Could you check a few things on this drawing? It's one solid part, dimensions in mm from its lowest x, y, z. A direction names the side the tool comes from. Coordinates: 2 decimals unless noted, no trailing zeros. Write each loop counter-clockwise with the first axis right and the second up, starting at its lowest first coordinate (ties: lowest second). Pieces come first, ordered by that corner, then holes. Notation, with made-up numbers: M -25,61 L 7,61 A15 ccw 7,85 Z; hole C -13.75,-22 d11. An arc over 180 degrees is marked long. Use a Markdown table: item, result.
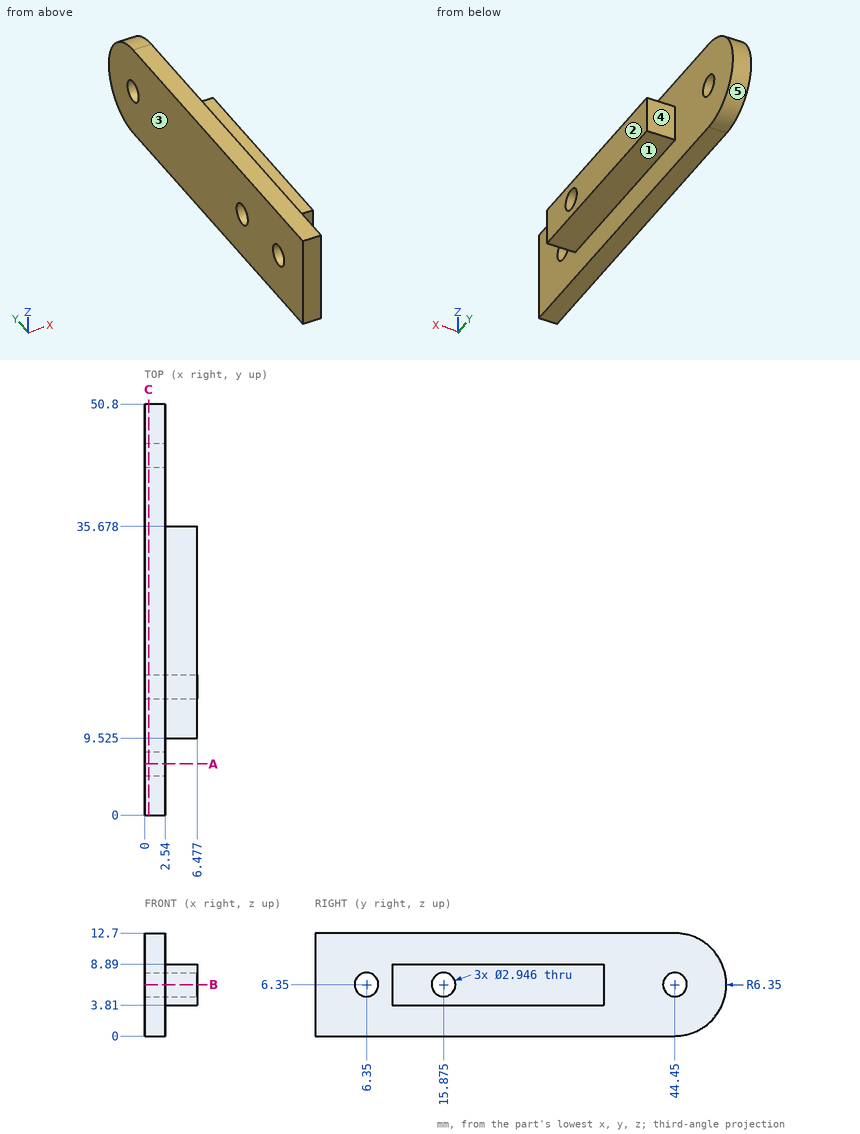
1. Which directions (+Z, -Z, +X, -X, +Y, -Y) give clear straight access to the entire face, cutting with the end or side of a thin tool? Please do the marked faces 4 and 5.
Answers follow:
| item | result |
|---|---|
| face 4 | +Z, -Z, +X, +Y |
| face 5 | +X, -X, +Y |
2. Will these pins go through, and if not, where does the flat tip stop? pin 1 Ø3 at (y, z) = (37.5, 9) entering from +X; pin 2 Ø2.5 at (y, z) = (15.875, 6.35) entering from +X; pin 3 Ø3 at (x, y) = (5, 22) entering from +Z; pin 4 Ø1.5 at (x, z) = (1, 5) entering from -Y.
Answers follow:
| item | result |
|---|---|
| pin 1 | stops at x = 2.54 |
| pin 2 | passes through |
| pin 3 | stops at z = 8.89 |
| pin 4 | stops at y = 0 |
3. I need wall thicknesses on probe 1 along Y at (x, z) = (0.8, 6.35); probe 2 along Y at (x, z) = (4.75, 6.35) (1 decimal); probe 3 along Z at (x, y) = (5, 18). Which ranges of each line are inside material? Lowest first, please.
Answers follow:
| item | result |
|---|---|
| probe 1 | y = 0 to 4.88, 7.82 to 14.4, 17.35 to 42.98, 45.92 to 50.8 |
| probe 2 | y = 9.5 to 14.4, 17.3 to 35.7 |
| probe 3 | z = 3.81 to 8.89 |
4. We'd pull the mould along X, two halves only. Please class the marked faces 1, 2 and 3: +X half, -X half, draft (parallel to the pull), parting line (faces both ways), or undercut.
Answers follow:
| item | result |
|---|---|
| face 1 | draft |
| face 2 | +X half |
| face 3 | -X half |
5. Suppose I cut it at B-B on z = 6.35. Write out the boundary of the cut face in (x, y) (1 decimal).
Answers follow:
| item | result |
|---|---|
| outline | M 0,0 L 2.5,0 L 2.5,4.9 L 0,4.9 Z; M 0,7.8 L 2.5,7.8 L 2.5,9.5 L 6.5,9.5 L 6.5,14.4 L 0,14.4 Z; M 0,17.3 L 6.5,17.3 L 6.5,35.7 L 2.5,35.7 L 2.5,43 L 0,43 Z; M 0,45.9 L 2.5,45.9 L 2.5,50.8 L 0,50.8 Z |
6. Suppose I cut it at A-A on y = 6.35. Write out the boundary of the cut face in (x, z).
Answers follow:
| item | result |
|---|---|
| outline | M 0,0 L 2.54,0 L 2.54,4.88 L 0,4.88 Z; M 0,7.82 L 2.54,7.82 L 2.54,12.7 L 0,12.7 Z |
7. Suppose I cut it at C-C on x = 0.5. State how many separate pieces and enclosed holes the cut face has.
Answers follow:
| item | result |
|---|---|
| separate pieces | 1 |
| enclosed holes | 3 |
